Could you check a few things on this model? Use its own coordinates, in mm. A direction names the side the tool comes from. Give positions to 0.01 mm unless a question says otherwise; leave off trailing zeros. Loops run counter-clockwise (first coordinate to the right, second up) from the corner with the lowest first, then second, coordinate; pieces in that order, holes last. Notation, with made-up numbers: M -40,13 L 16,13 A37 ccw 16,50 Z; hole C 24,13 d6. An arc over 180 degrees is marked long. Answer in a Markdown table with one row per item. Add a question column.
```python
from build123d import *

# Parameters (mm, degrees)
SKETCH1_R           = 1.6
BOSS_EXTRUDE1_DEPTH = 3
SKETCH2_R           = 3.5
SKETCH2_R_2         = 1.6
BOSS_EXTRUDE2_DEPTH = 3


with BuildPart() as part:
    # Sketch1 → Boss-Extrude1 (new body)
    with BuildSketch(Plane(origin=(0, 0, 0), x_dir=(1, 0, 0), z_dir=(0, 1, 0))):
        Polygon((0, 7.54), (90.17, 7.54), (90.17, 45.8), (0, 45.8), (0, 55.8), (100.17, 55.8), (100.17, -2.46), (0, -2.46), align=None)
        with Locations((15.24, 2.54)):
            Circle(SKETCH1_R, mode=Mode.SUBTRACT)
        with Locations((96.52, 2.54)):
            Circle(SKETCH1_R, mode=Mode.SUBTRACT)
        with Locations((15.24, 50.8)):
            Circle(SKETCH1_R, mode=Mode.SUBTRACT)
        with Locations((90.17, 50.8)):
            Circle(SKETCH1_R, mode=Mode.SUBTRACT)
    extrude(amount=BOSS_EXTRUDE1_DEPTH)

    # Sketch2 → Boss-Extrude2 (add)
    with BuildSketch(Plane(origin=(0, 3, 0), x_dir=(1, 0, 0), z_dir=(0, 1, 0))):
        with Locations((15.24, 50.8)):
            Circle(SKETCH2_R)
        with Locations((15.24, 50.8)):
            Circle(SKETCH2_R_2, mode=Mode.SUBTRACT)
        with Locations((90.17, 50.8)):
            Circle(SKETCH2_R)
        with Locations((90.17, 50.8)):
            Circle(SKETCH2_R_2, mode=Mode.SUBTRACT)
        with Locations((96.52, 2.54)):
            Circle(SKETCH2_R)
        with Locations((96.52, 2.54)):
            Circle(SKETCH2_R_2, mode=Mode.SUBTRACT)
        with Locations((15.24, 2.54)):
            Circle(SKETCH2_R)
        with Locations((15.24, 2.54)):
            Circle(SKETCH2_R_2, mode=Mode.SUBTRACT)
    extrude(amount=BOSS_EXTRUDE2_DEPTH)


solid = part.part
```
Item 1: Suppose I cut it at A-A (x = 49). List the corners of the cut face in (y, z) for me, then the cut area to 3 significant figures.
Item 2: For faces 1 (the face through (90.17, 1, -26)), 2 (the face through (92, 6, -50)), 3 (the face through (91.785, 4.479, -47.695)), which set-ups out of +Z, -Z, +X, -X, +Y, -Y let a thin tool reach every point of the face, with its end or its side?
Item 3: I need wall thicknesses on L1, parallel to Z at x = 15.24, y = 2.95; L2, parallel to Z at x = 15, y = 5.65; L3, parallel to X at y = 4.2, z = -2.54. Which ranges of each line are inside material? Lowest first, please.
Item 4: Suppose I cut it at B-B (y = 4.15). List the corners of the cut face in (x, z) for me, then the cut area to 3 significant figures.
Item 5: For P1, Ø1.5, axis at y = 1.5, z = -20, coming from the -X side, with a flat end and sliding along its axis, tell me the tip position at first contact or that it passes through.
Item 6: Suppose I cut it at C-C (z = -2.54). List the corners of the cut face in (x, y) for me, then the cut area to 3 significant figures.
Item 7: Suppose I cut it at D-D (x = 15.24). List the corners of the cut face in (y, z) for me.
Item 8: If we mould it in two halves opening along Z, with no side actions, what happens to faces 4 (the face through (17, 6, -2)), 5 (the face through (49, 1, -55.8)), 6 (the face through (13.97, 2.96, -1.57)), 7 (the face through (98, 2.96, -1.93))? For each: +Z half, -Z half, draft (parallel to the pull), parting line (faces both ways), or undercut.
Values found:
| question | item | result |
|---|---|---|
| 1 | outline | M 0,-55.8 L 3,-55.8 L 3,-45.8 L 0,-45.8 Z; M 0,-7.54 L 3,-7.54 L 3,2.46 L 0,2.46 Z |
| 1 | area | 60.0 mm² |
| 2 | face 1 | -X, +Y, -Y |
| 2 | face 2 | +Z, -Z, +X, -X, +Y |
| 2 | face 3 | +Y |
| 3 | L1 | -55.8 to -52.4, -49.2 to -45.8, -7.54 to -4.14, -0.94 to 2.46 |
| 3 | L2 | -54.29 to -52.38, -49.22 to -47.31, -6.03 to -4.12, -0.96 to 0.95 |
| 3 | L3 | 11.74 to 13.64, 16.84 to 18.74, 93.02 to 94.92, 98.12 to 100.02 |
| 4 | outline | C 15.24,-50.8 d7; C 15.24,-2.54 d7; C 90.17,-50.8 d7; C 96.52,-2.54 d7; hole C 15.24,-50.8 d3.2; hole C 15.24,-2.54 d3.2; hole C 90.17,-50.8 d3.2; hole C 96.52,-2.54 d3.2 |
| 4 | area | 122 mm² |
| 5 | P1 | x = 90.17 |
| 6 | outline | M 0,0 L 13.64,0 L 13.64,6 L 11.74,6 L 11.74,3 L 0,3 Z; M 16.84,0 L 94.92,0 L 94.92,6 L 93.02,6 L 93.02,3 L 18.74,3 L 18.74,6 L 16.84,6 Z; M 98.12,0 L 100.17,0 L 100.17,3 L 100.02,3 L 100.02,6 L 98.12,6 Z |
| 6 | area | 304 mm² |
| 7 | outline | M 0,-55.8 L 3,-55.8 L 3,-54.3 L 6,-54.3 L 6,-52.4 L 0,-52.4 Z; M 0,-49.2 L 6,-49.2 L 6,-47.3 L 3,-47.3 L 3,-45.8 L 0,-45.8 Z; M 0,-7.54 L 3,-7.54 L 3,-6.04 L 6,-6.04 L 6,-4.14 L 0,-4.14 Z; M 0,-0.94 L 6,-0.94 L 6,0.96 L 3,0.96 L 3,2.46 L 0,2.46 Z |
| 8 | face 4 | draft |
| 8 | face 5 | -Z half |
| 8 | face 6 | undercut |
| 8 | face 7 | undercut |
